Here's how the part is built. I have some questions about the finished solid (model axes, mm). A direction names the side the tool comes from. Round coordinates to 2 decimals unless told otherwise and drop trailing zeros. Order: outer loops, then holes, each group sorted by start corner. A loop starts at its lowest first (then second) coordinate and runs counter-clockwise, first axis right, second up. Notation, with made-up numbers: M 78.5,78.5 L 101.5,78.5 A20 cw 101.5,103.5 Z; hole C 55.5,86 d4. An arc over 180 degrees is marked long. Write each question's results on one line, items separated by ' | '. Start each with the question number.
```python
from build123d import *

# Parameters (mm, degrees)
SKETCH1_R           = 10
BOSS_EXTRUDE1_DEPTH = 10
BOSS_EXTRUDE2_DEPTH = 10
SKETCH3_W           = 10
SKETCH3_H           = 10
BOSS_EXTRUDE3_DEPTH = 10


with BuildPart() as part:
    # Sketch1 → Boss-Extrude1 (new body)
    with BuildSketch(Plane(origin=(0, 0, 0), x_dir=(1, 0, 0), z_dir=(0, 1, 0))):
        with BuildLine():
            Line((-27.984790875, 21.292775665), (-27.984790875, -18.707224335))
            Line((-27.984790875, -18.707224335), (-7.984790875, -18.436045575))
            ThreePointArc((-7.984790875, -18.436045575), (5.96559241, -12.657607619), (11.744030366, 1.292775665))
            Line((11.744030366, 1.292775665), (12.015209125, 21.292775665))
            Line((12.015209125, 21.292775665), (-27.984790875, 21.292775665))
        make_face()
        with Locations(Location((-7.984790875, 1.292775665, 0), (0, 0, 270))):
            Circle(SKETCH1_R, mode=Mode.SUBTRACT)
    extrude(amount=BOSS_EXTRUDE1_DEPTH)

    # Sketch2 → Boss-Extrude2 (add)
    with BuildSketch(Plane.ZY.offset(27.984790875)):
        Polygon((18.707224335, 10), (8.707224335, 20), (-1.292775665, 20), (-11.292775665, 30), (-21.292775665, 30), (-21.292775665, 10), align=None)
    extrude(amount=-BOSS_EXTRUDE2_DEPTH)

    # Sketch3 → Boss-Extrude3 (add)
    with BuildSketch(Plane(origin=(0, 0, -21.292775665), x_dir=(-1, 0, 0), z_dir=(0, 0, -1))):
        Polygon((17.984790875, 30), (17.984790875, 10), (7.984790875, 10), (7.984790875, 20), align=None)
        with Locations((-7.015209125, 15)):
            Rectangle(SKETCH3_W, SKETCH3_H)
    extrude(amount=-BOSS_EXTRUDE3_DEPTH)


solid = part.part
```
(1) I'm going to push flat-ended pins straight in: pin 1 Ø10 at (y, z) = (8.5, 9.5) entering from +X; pin 2 Ø10 at (x, z) = (-2, -16) entering from +Y; pin 3 Ø3 at (x, y) = (6.5, 16.5) entering from +Z; pin 4 Ø18 at (x, z) = (-7.98, -1.29) entering from -Y. Where does each tip first touch, or does it pass through?
(2) On a 3-axis mill with a long thin cutter (end or side, diameter ignored), from which of +Z, -Z, +X, -X, +Y, -Y can I reach the whole of each face in a straight line? I mean faces 1 (the flat face through (-23, 20, 4)), 2 (the flat face through (-7.985, 15, -16)), 3 (the flat face through (-16, 10, -9)). Say none if no direction works.
(3) If we mould it in two halves opening along X, with no side actions, what happens to faces 4 (the flat face through (7, 15, -11.293)), 5 (the flat face through (-17.985, 16, 0)), 6 (the flat face through (3, 10, 3)), 7 (the flat face through (2.015, 15, -16))? For each: pulls with the +X half, pulls with the -X half, needs draft (parallel to the pull), parting line crosses it, or undercut.
(4) Please list where these lines run through material, in increasing order: line 1 (Y direction, x = -15, z = 7.5); line 2 (X direction, y = 16.75, z = -14); line 3 (Z direction, x = -13, y = 21.5).
(5) I want a section at B-B on x = -13. Write out the boundary of the cut face in (y, z).
(6) I want a section at C-C on y = 6.5. Write out the boundary of the cut face in (x, z).
(7) I want a section at D-D on x = -25. Write out the boundary of the cut face in (y, z), and give its area (3 significant figures).
Solutions:
1) pin 1: x = 10.87 | pin 2: y = 20 | pin 3: z = -11.29 | pin 4: through
2) face 1: +Z, +X, -X, +Y | face 2: +Z, -Z, +Y | face 3: +Z, +X, +Y
3) face 4: needs draft | face 5: pulls with the +X half | face 6: undercut | face 7: undercut
4) line 1: 0 to 10 | line 2: -27.98 to -7.98, 2.02 to 12.02 | line 3: -21.29 to -11.29
5) outline: M 0,-21.29 L 25.02,-21.29 L 25.02,-11.29 L 10,-11.29 L 10,-9.94 L 0,-9.94 Z; M 0,7.36 L 10,7.36 L 10,18.5 L 0,18.5 Z
6) outline: M -27.98,-21.29 L 12.02,-21.29 L 11.74,-1.29 A19.73 ccw -7.98,18.44 L -27.98,18.71 Z; hole C -7.98,-1.29 d20
7) outline: M 0,-21.29 L 30,-21.29 L 30,-11.29 L 20,-1.29 L 20,8.71 L 10,18.71 L 10,18.67 L 0,18.67 Z | area: 900 mm^2
